Can you work these out from the model? Positions are in its coordinate system, mm. Give positions to 0.01 mm unless a question says otherwise; leave off trailing zeros. Write each loop counter-clockwise with the first axis right and the second up, starting at its lowest first coordinate (ties: lowest second). Pieces come first, ordered by that corner, then holes. Notation, with made-up numbers: M -9,71.25 L 1,71.25 A10 cw 1,83.25 Z; hole C 43.5,-26.75 d2. An arc over 180 degrees is marked long. Write each question's results on one line, items separated by ' | '.
from build123d import *

# Parameters (mm, degrees)
CYLINDER005_R     = 2
CYLINDER005_DEPTH = 2
CYLINDER006_R     = 2
CYLINDER006_DEPTH = 2
CYLINDER004_R     = 2
CYLINDER004_DEPTH = 2
CYLINDER003_R     = 2
CYLINDER003_DEPTH = 2
CYLINDER022_R     = 11
CYLINDER022_DEPTH = 2
CYLINDER023_R     = 4
CYLINDER023_DEPTH = 2
CYLINDER002_R     = 39.25
CYLINDER002_DEPTH = 2
BOX002_W          = 80
BOX002_H          = 117
BOX002_DEPTH      = 2


with BuildPart() as mounthole002:
    # Cylinder005 → Cylinder005 (new body)
    with BuildSketch(Plane(origin=(63, 63, 20), x_dir=(1, 0, 0), z_dir=(0, 0, 1))):
        Circle(CYLINDER005_R)
    extrude(amount=CYLINDER005_DEPTH)


with BuildPart() as mounthole003:
    # Cylinder006 → Cylinder006 (new body)
    with BuildSketch(Plane(origin=(0, 63, 20), x_dir=(1, 0, 0), z_dir=(0, 0, 1))):
        Circle(CYLINDER006_R)
    extrude(amount=CYLINDER006_DEPTH)


with BuildPart() as mounthole001:
    # Cylinder004 → Cylinder004 (new body)
    with BuildSketch(Plane(origin=(63, 0, 20), x_dir=(1, 0, 0), z_dir=(0, 0, 1))):
        Circle(CYLINDER004_R)
    extrude(amount=CYLINDER004_DEPTH)


with BuildPart() as mountholes:
    # Cylinder003 → Cylinder003 (new body)
    with BuildSketch(Plane.XY.offset(20)):
        Circle(CYLINDER003_R)
    extrude(amount=CYLINDER003_DEPTH)

    # Fusion: union MountHole002, MountHole003, MountHole001
    add(mounthole002.part)
    add(mounthole003.part)
    add(mounthole001.part)


with BuildPart() as mountholes_1:
    # Fusion placement: moved
    add(mountholes.part.moved(Location((6.5, 6.5, 0))))


with BuildPart() as mounttubehole:
    # Cylinder022 → Cylinder022 (new body)
    with BuildSketch(Plane(origin=(15, -20, 20), x_dir=(1, 0, 0), z_dir=(0, 0, 1))):
        Circle(CYLINDER022_R)
    extrude(amount=CYLINDER022_DEPTH)


with BuildPart() as volumehole001:
    # Cylinder023 → Cylinder023 (new body)
    with BuildSketch(Plane(origin=(62, -19, 20), x_dir=(1, 0, 0), z_dir=(0, 0, 1))):
        Circle(CYLINDER023_R)
    extrude(amount=CYLINDER023_DEPTH)


with BuildPart() as obj1:
    # Cylinder002 → Cylinder002 (new body)
    with BuildSketch(Plane(origin=(38, 38, 20), x_dir=(1, 0, 0), z_dir=(0, 0, 1))):
        Circle(CYLINDER002_R)
    extrude(amount=CYLINDER002_DEPTH)

    # Fusion001: union MountHoles, MountTubeHole, VolumeHole001
    add(mountholes_1.part)
    add(mounttubehole.part)
    add(volumehole001.part)


with BuildPart() as mount:
    # Box002 → Box002 (new body)
    with BuildSketch(Plane(origin=(-2, -39, 20), x_dir=(1, 0, 0), z_dir=(0, 0, 1))):
        with Locations((40, 58.5)):
            Rectangle(BOX002_W, BOX002_H)
    extrude(amount=BOX002_DEPTH)

    # Cut013: cut obj1
    add(obj1.part, mode=Mode.SUBTRACT)


with BuildPart() as mount_1:
    # Cut013 placement: moved
    add(mount.part.moved(Location((0, 2, 0))))


solid = mount_1.part
Item 1: Thinking about a two-plate mould opening in X: for faces 1 (the face through (12.62, -28.74, 20.99)), 2 (the face through (37, -4, 20)), which applies, +X half, -X half, draft (parallel to the pull), parting line (faces both ways), or undercut?
Geometry says:
face 1: undercut | face 2: draft
Item 2: If I drill on line 1 (Y direction, x = 6.5, z = 20.85); line 2 (Y direction, x = 69.5, z = 21); line 3 (Y direction, x = 69, z = 21.5), over which ranges is the centre line in solid material (lowest first)? Write a range as from..to.
Geometry says:
line 1: y = -37..-24.98, -11.02..6.5, 10.5..16.58, 63.42..69.5, 73.5..80 | line 2: y = -37..6.5, 10.5..16.58, 63.42..69.5, 73.5..80 | line 3: y = -37..6.56, 10.44..15.93, 64.07..69.56, 73.44..80
Item 3: I want a section at A-A, the plane x = 38. Please give me the cut outline in (y, z), and give its area (3 significant figures).
Geometry says:
outline: M -37,20 L 0.75,20 L 0.75,22 L -37,22 Z; M 79.25,20 L 80,20 L 80,22 L 79.25,22 Z | area: 77.0 mm2
Item 4: I want a section at D-D, the plane x = 69.5. Please give me the cut outline in (y, z).
Geometry says:
outline: M -37,20 L 6.5,20 L 6.5,22 L -37,22 Z; M 10.5,20 L 16.58,20 L 16.58,22 L 10.5,22 Z; M 63.42,20 L 69.5,20 L 69.5,22 L 63.42,22 Z; M 73.5,20 L 80,20 L 80,22 L 73.5,22 Z
Item 5: I'm going to push flat-ended pins straight in: pin 1 (2.5 mm diameter, centred on x = 6.5, y = 8.5, fed in from -Z); pin 2 (5 mm diameter, centred on x = 6.5, y = 71.5, fed in from +Z). Where does each tip first touch, or does it pass through?
Geometry says:
pin 1: passes through | pin 2: stops at z = 22
Item 6: I want a section at B-B, the plane y = 40. Please give me the cut outline in (x, z).
Geometry says:
outline: M -2,20 L -1.25,20 L -1.25,22 L -2,22 Z; M 77.25,20 L 78,20 L 78,22 L 77.25,22 Z
Item 7: I want a section at C-C, the plane z = 21.15. Please give me the cut outline in (x, y), and give its area (3 significant figures).
Geometry says:
outline: M -2,-37 L 78,-37 L 78,80 L -2,80 Z; hole C 38,40 d78.5; hole C 15,-18 d22; hole C 6.5,8.5 d4; hole C 6.5,71.5 d4; hole C 62,-17 d8; hole C 69.5,8.5 d4; hole C 69.5,71.5 d4 | area: 4,040 mm2
